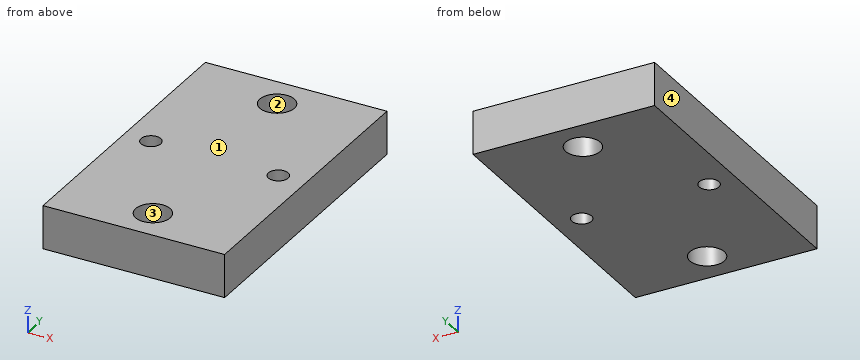
```python
from build123d import *

# Parameters (mm, degrees)
SKETCH1_W           = 21
SKETCH1_H           = 34
BOSS_EXTRUDE1_DEPTH = 5
SKETCH2_R           = 1.143
CUT_EXTRUDE1_DEPTH  = 10
SKETCH3_R           = 2
CUT_EXTRUDE2_DEPTH  = 10


with BuildPart() as part:
    # Sketch1 → Boss-Extrude1 (new body)
    with BuildSketch(Plane.XY):
        Rectangle(SKETCH1_W, SKETCH1_H)
    extrude(amount=BOSS_EXTRUDE1_DEPTH)

    # Sketch2 → Cut-Extrude1 (cut)
    with BuildSketch(Plane(origin=(0, 0, 0), x_dir=(-1, 0, 0), z_dir=(0, 0, -1))):
        with Locations((7.411509934, 0)):
            Circle(SKETCH2_R)
        with Locations((-7.320490066, 0)):
            Circle(SKETCH2_R)
    extrude(amount=-CUT_EXTRUDE1_DEPTH, mode=Mode.SUBTRACT)

    # Sketch3 → Cut-Extrude2 (cut)
    with BuildSketch(Plane(origin=(0, 0, 0), x_dir=(-1, 0, 0), z_dir=(0, 0, -1))):
        with Locations((0, -13)):
            Circle(SKETCH3_R)
        with Locations((0, 13)):
            Circle(SKETCH3_R)
    extrude(amount=-CUT_EXTRUDE2_DEPTH, mode=Mode.SUBTRACT)


solid = part.part
```
Can you work these out from the model? Positions are in its coordinate system, mm. Face numbers are marked on the shaded views. Give positions to 0.01 mm unless a question says otherwise; leave off trailing zeros. Order: outer loops, then holes, each group sorted by start corner. A loop starts at its lowest first (then second) coordinate and runs counter-clockwise, first axis right, second up. Notation, with made-up numbers: (31, -37.75) - (74, -37.75) arc R16 cw to (74, -21.75) - close; hole circle Ø10 at (76, 14). An arc over 180 degrees is marked (long way). Use a Markdown table: item, result. Add a question column.
Q1. If we mould it in two halves opening along X, with no side actions, what happens to the marked faces 1, 2, 3 and 4? For each: released by +X, released by -X, zero draft, split by the parting line, or undercut.
Q2. If we section it at A-A on y = 0: Write out the boundary of the cut face in (x, z), plus the area to 3 significant figures.
Q3. If we section it at D-D on x = 0: Write out the boundary of the cut face in (y, z), plus the area to 3 significant figures.
Q4. If we section it at C-C on y = 13: Write out the boundary of the cut face in (x, z).
Q5. I'm going to push a flat-ended pin straight in: pin 1 (1.8 mm diameter, centred on x = -7.41, y = 0, fed in from -Z). Where does the tip first touch, or does it pass through?
Q6. If we section it at B-B on z = 1.55: Write out the boundary of the cut face in (x, y).
Q7. Please list where these lines run through material, in increasing order: line 1 along Y through (x, z) = (0.5, 1); line 2 along Y through (x, z) = (7, 4.15); line 3 along X through (y, z) = (-14, 1.6).
Answers follow:
| question | item | result |
|---|---|---|
| 1 | face 1 | zero draft |
| 1 | face 2 | undercut |
| 1 | face 3 | undercut |
| 1 | face 4 | released by -X |
| 2 | outline | (-10.5, 0) - (-8.55, 0) - (-8.55, 5) - (-10.5, 5) - close; (-6.27, 0) - (6.18, 0) - (6.18, 5) - (-6.27, 5) - close; (8.46, 0) - (10.5, 0) - (10.5, 5) - (8.46, 5) - close |
| 2 | area | 82.1 mm^2 |
| 3 | outline | (-17, 0) - (-15, 0) - (-15, 5) - (-17, 5) - close; (-11, 0) - (11, 0) - (11, 5) - (-11, 5) - close; (15, 0) - (17, 0) - (17, 5) - (15, 5) - close |
| 3 | area | 130 mm^2 |
| 4 | outline | (-10.5, 0) - (-2, 0) - (-2, 5) - (-10.5, 5) - close; (2, 0) - (10.5, 0) - (10.5, 5) - (2, 5) - close |
| 5 | pin 1 | passes through |
| 6 | outline | (-10.5, -17) - (10.5, -17) - (10.5, 17) - (-10.5, 17) - close; hole circle Ø2.29 at (-7.41, 0); hole circle Ø4 at (0, -13); hole circle Ø4 at (0, 13); hole circle Ø2.29 at (7.32, 0) |
| 7 | line 1 | y = -17 to -14.94, -11.06 to 11.06, 14.94 to 17 |
| 7 | line 2 | y = -17 to -1.1, 1.1 to 17 |
| 7 | line 3 | x = -10.5 to -1.73, 1.73 to 10.5 |
